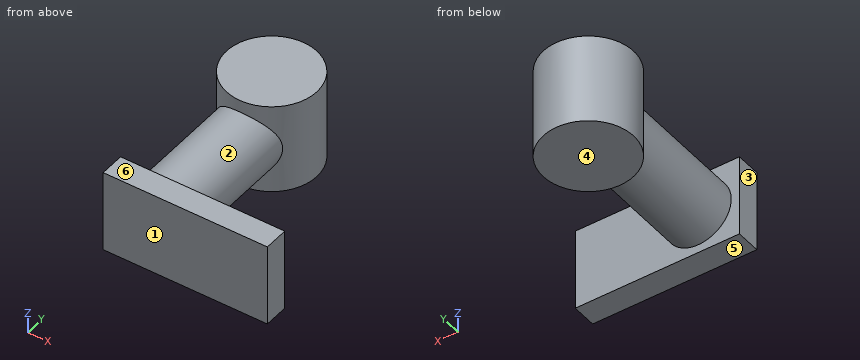
```python
from build123d import *

# Parameters (mm, degrees)
SKETCH1_R           = 40
BOSS_EXTRUDE1_DEPTH = 190
SKETCH2_R           = 55
BOSS_EXTRUDE2_DEPTH = 55
SKETCH3_W           = 200
SKETCH3_H           = 100
BOSS_EXTRUDE3_DEPTH = 30


with BuildPart() as part:
    # Sketch1 → Boss-Extrude1 (new body)
    with BuildSketch(Plane(origin=(0, 0, 0), x_dir=(1, 0, 0), z_dir=(0, 1, 0))):
        with Locations(Location((0, 0, 0), (0, 0, 270))):
            Circle(SKETCH1_R)
    extrude(amount=BOSS_EXTRUDE1_DEPTH)

    # Sketch2 → Boss-Extrude2 (add, symmetric)
    with BuildSketch(Plane.XY):
        with Locations((0, 190)):
            Circle(SKETCH2_R)
    extrude(amount=BOSS_EXTRUDE2_DEPTH, both=True)

    # Sketch3 → Boss-Extrude3 (add)
    with BuildSketch(Plane.XZ):
        with Locations((50, 0)):
            Rectangle(SKETCH3_W, SKETCH3_H)
    extrude(amount=BOSS_EXTRUDE3_DEPTH)


solid = part.part
```
Could you check a few things on this model? Use its own coordinates, in mm. Face numbers are marked on the shaded views. A direction names the side the tool comes from. Give positions to 0.01 mm unless a question says otherwise; leave off trailing zeros. Write each loop counter-clockwise with the first axis right and the second up, starting at its lowest first coordinate (ties: lowest second). Pieces come first, ordered by that corner, then holes. Notation, with made-up numbers: (1, 0.5) -> (36, 0.5) arc R8 cw to (36, 9.5) -> close; hole circle Ø4 at (56.25, 87.5). An arc over 180 degrees is marked (long way). Write each question's results on one line, items separated by ' | '.
1. On a 3-axis mill with a long thin cutter (end or side, diameter ignored), from which of +Z, -Z, +X, -X, +Y, -Y can I reach the whole of each face in a straight line? I mean the marked faces 4, 5 and 6. Say none if no direction works.
Check sheet entries:
face 4: -Z, +X, -X, +Y, -Y | face 5: -Z, +X, -X, -Y | face 6: +Z, +X, -X, -Y
2. I want a section at B-B, the plane x = 0. Write out the boundary of the cut face in (y, z), then the cut area to 3 significant figures.
Check sheet entries:
outline: (-30, -50) -> (0, -50) -> (0, -40) -> (135, -40) -> (135, -55) -> (245, -55) -> (245, 55) -> (135, 55) -> (135, 40) -> (0, 40) -> (0, 50) -> (-30, 50) -> close | area: 25,900 mm²
3. If we mould it in two halves opening along Y, with no side actions, what happens to the marked faces 1, 2 and 3? For each: released by +Y, released by -Y, zero draft, split by the parting line, or undercut.
Check sheet entries:
face 1: released by -Y | face 2: undercut | face 3: zero draft
4. I want a section at D-D, the plane x = 31. Write out the boundary of the cut face in (y, z).
Check sheet entries:
outline: (-30, -50) -> (0, -50) -> (0, -25.28) -> (144.57, -25.28) -> (144.57, -55) -> (235.43, -55) -> (235.43, 55) -> (144.57, 55) -> (144.57, 25.28) -> (0, 25.28) -> (0, 50) -> (-30, 50) -> close
5. Will these pins go through, and if not, where does the flat tip stop? pin 1 Ø24 at (y, z) = (-20, 2) entering from -X; pin 2 Ø1.5 at (y, z) = (106.5, 7.5) entering from -X; pin 3 Ø6 at (y, z) = (36, -23.5) entering from -X.
Check sheet entries:
pin 1: stops at x = -50 | pin 2: stops at x = -39.43 | pin 3: stops at x = -34.35
6. I need wall thicknesses on L1, parallel to Y at x = 1, z = 46; L2, parallel to Y at x = 115, z = 3; L3, parallel to Y at x = 44.5, z = -34. Which ranges of each line are inside material? Lowest first, please.
Check sheet entries:
L1: y = -30 to 0, 135.01 to 244.99 | L2: y = -30 to 0 | L3: y = -30 to 0, 157.68 to 222.32
7. I want a section at C-C, the plane y = 190. Write out the boundary of the cut face in (x, z), then the cut area to 3 significant figures.
Check sheet entries:
outline: (-55, -55) -> (55, -55) -> (55, 55) -> (-55, 55) -> close | area: 12,100 mm²
8. I want a section at A-A, the plane z = 0. Write out the boundary of the cut face in (x, y), then the cut area to 3 significant figures.
Check sheet entries:
outline: (-50, -30) -> (150, -30) -> (150, 0) -> (40, 0) -> (40, 152.25) arc R55 ccw (long way) to (-40, 152.25) -> (-40, 0) -> (-50, 0) -> close | area: 26,700 mm²
